Source: CAD feature listing. Evaluate the final solid. Frame: model axes, mm. A direction names the side the tool comes from. Round coordinates to 2 decimals unless told otherwise and drop trailing zeros. Write each loop counter-clockwise with the first axis right and the second up, starting at its lowest first coordinate (ties: lowest second). Pieces come first, ordered by that corner, then holes. Notation, with made-up numbers: M 65.25,71.5 L 108.25,71.5 A27 ccw 108.25,104.5 Z; hole C -29.75,60.25 d5. An arc over 180 degrees is marked long. Answer in a Markdown table with one row per item. Add a question column.
Item 1: Cut plane B-B on z = 96. Return loops of the section in (x, y), and give its area (3 significant figures).
Item 2: Set-up query: faces 1 (the face through (5, 0, 5)), 2 (the face through (-11, 1, 5)), 3 (the face through (-10.95, 5.6, 9.43)). Return all of +Z, -Z, +X, -X, +Y, -Y with unobstructed straight access to the full face (end or side cutting, diameter ignored); none if empty.
Item 3: Cut plane A-A on x = -8. Return loops of the section in (y, z).
Item 4: Mould query, pull axis Y, two halves, no side actions, for faces 4 (the face through (-11, 6.2, 5)), 5 (the face through (-1, 4, 57)), 6 (the face through (-0.57, 12.13, 9.4)). Classes: released by +Y, released by -Y, zero draft, split by the parting line, or undercut.
Item 5: Contact query for flat-ended pins moving along their axis: pin 1 (6 mm diameter, centred on x = -4, z = 49, fed in from -Y); pin 2 (3 mm diameter, centred on x = -10.5, y = 11.5, fed in from +Z); pin 3 (2.5 mm diameter, centred on y = 3.5, z = 81, fed in from -X). Output: stop coordinate, or through.
Item 6: Cut plane C-C on y = -6.75. Return loops of the section in (x, z).
Item 7: Material intervals for probe 1 along Z at (x, y) = (-8, 12.25); probe 2 along X at (y, z) = (5.5, 86); probe 3 along Y at (x, z) = (-4, 59.5), sorted ascending.
Autodesk Inventor part; units mm, degrees
ref_plane "YZ Plane" through (0, 0, 0) normal (1, 0, 0) x (0, 1, 0)
ref_plane "XZ Plane" through (0, 0, 0) normal (0, 1, 0) x (-1, 0, 0)
ref_plane "XY Plane" through (0, 0, 0) normal (0, 0, 1) x (1, 0, 0)
sketch "Esboço1" plane through (0, 0, 0) normal (0, 0, 1) x (1, 0, 0)
  point P0 (0, 0)
sketch "Esboço2" plane through (0, 0, 0) normal (0, 0, 1) x (1, 0, 0)
  line L0 (0, 0) -> (0, 7.2)
  line L1 (0, 7.2) -> (-5.75, 7.2)
  line L2 (-5.75, 7.2) -> (-5.75, 6.2)
  line L3 (-5.75, 6.2) -> (-1, 6.2)
  line L4 (-1, 6.2) -> (-1, 1)
  line L5 (0, 0) -> (-5.75, 0)
  line L6 (-5.75, 0) -> (-5.75, 1)
  line L7 (-5.75, 1) -> (-1, 1)
  dimension "d0" = 7.2
  dimension "d1" = 1
  dimension "d2" = 5.75
  dimension "d3" = 4.75
  dimension "d4" = 5.2
extrude "Extrusão1" add sketch "Esboço2" along normal blind 105
sketch "Esboço3" plane through (-5.75, 0, 0) normal (0, -1, 0) x (1, 0, 0)
  line L0 (5.75, 0) -> (5.75, 105)
  line L1 (5.75, 0) -> (5.75, 10)
  line L2 (5.75, 10) -> (0, 10)
  line L3 (0, 0) -> (0, 105)
  line L4 (0, 10) -> (0, 0)
  line L5 (0, 0) -> (5.75, 0)
  line L6 (0, 0) -> (5.75, 0)
  dimension "d7" = 10
extrude "Extrusão2" add sketch "Esboço3" along normal blind 10
sketch "Esboço4" plane through (0, 0, 105) normal (1, 0, 0) x (0, 0, -1)
  line L0 (105, -10) -> (105, 7.2)
  line L1 (105, 0) -> (105, 7.2)
  line L2 (95, 0) -> (95, -10)
  line L3 (105, 0) -> (95, 0)
  line L4 (95, 0) -> (95, 7.2)
  line L5 (105, 7.2) -> (0, 7.2)
  line L6 (95, 7.2) -> (105, 7.2)
extrude "Extrusão3" add sketch "Esboço4" along normal blind 10
sketch "Esboço5" plane through (-5.75, 7.2, 105) normal (0, 1, 0) x (1, 0, 0)
  line L0 (0, 105) -> (5.75, 105)
  line L1 (0, 105) -> (15.75, 105)
  line L2 (5.75, 105) -> (5.75, 95)
  line L3 (5.75, 95) -> (5.75, 105)
  line L4 (5.75, 95) -> (5.75, 0)
  line L5 (5.75, 105) -> (5.75, 95)
  line L6 (5.75, 95) -> (0, 95)
  line L7 (0, 105) -> (0, 0)
  line L8 (0, 95) -> (0, 105)
extrude "Extrusão4" add sketch "Esboço5" along normal blind 10
sketch "Esboço6" plane through (0, 7.2, 10) normal (1, 0, 0) x (0, 0, -1)
  line L0 (10, -6.2) -> (10, -17.2)
  line L1 (10, -7.2) -> (0, -7.2)
  line L2 (10, -17.2) -> (7, -17.2)
  line L3 (7, -17.2) -> (7, -7.2)
  line L4 (7, -7.2) -> (10, -7.2)
  line L5 (10, -7.2) -> (10, -17.2)
  line L6 (10, -1) -> (10, 10)
  line L7 (10, 10) -> (0, 10)
  line L8 (10, 0) -> (7, 0)
  line L9 (7, 0) -> (7, 10)
  line L10 (7, 10) -> (10, 10)
  line L11 (10, 10) -> (10, 0)
  dimension "d14" = 3
extrude "Extrusão5" add sketch "Esboço6" along normal blind 10
fillet "Arredondamento1" radius 2 4 edges at (5, 7.2, 10) (0, 12.2, 10) (5, 0, 10) (0, -5, 10)
sketch "Esboço7" plane through (-1, 1, 0) normal (-1, 0, 0) x (0, 0, 1)
  line L0 (10, -1) -> (10, -11)
  line L1 (10, 16.2) -> (10, 6.2)
  line L2 (10, -1) -> (10, 6.2)
  line L3 (0, 0) -> (0, -11)
  line L4 (0, 5.2) -> (105, 5.2)
  line L5 (0, 0) -> (10, 0)
  line L6 (10, 0) -> (10, 5.2)
  line L7 (10, 5.2) -> (0, 5.2)
  line L8 (0, 5.2) -> (0, 0)
  point P0 (0, -1)
extrude "Extrusão6" add sketch "Esboço7" along normal blind 15
sketch "Esboço8" plane through (-5.75, 7.2, 10) normal (-1, 0, 0) x (0, 0, 1)
  line L0 (-10, 10) -> (0, 10)
  line L1 (-7, -7.2) -> (-7, -17.2)
  line L2 (-10, 10) -> (-7, 10)
  line L3 (-7, 10) -> (-7, -17.2)
  line L4 (-7, -17.2) -> (-10, -17.2)
  line L5 (-10, -17.2) -> (-10, 10)
  point P0 (-10, -7.2)
extrude "Extrusão7" add sketch "Esboço8" along normal blind 10.25
fillet "Arredondamento2" radius 2 4 edges at (-5.75, 12.2, 10) (-10.875, 6.2, 10) (-10.875, 1, 10) (-5.75, -5, 10)
properties part number "suporte para arma"
Results below:
| question | item | result |
|---|---|---|
| 1 | outline | M -5.75,0 L 0,0 L 0,7.2 L -5.75,7.2 L -5.75,6.2 L -1,6.2 L -1,1 L -5.75,1 Z |
| 1 | area | 16.7 mm2 |
| 2 | face 1 | +Z, +X, -Y |
| 2 | face 2 | +Z, -X, -Y |
| 2 | face 3 | +Z, -X, +Y |
| 3 | outline | M -10,0 L 17.2,0 L 17.2,3 L 6.2,3 L 6.2,8 A2 ccw 4.2,10 L 3,10 A2 ccw 1,8 L 1,3 L -10,3 Z |
| 4 | face 4 | released by +Y |
| 4 | face 5 | undercut |
| 4 | face 6 | zero draft |
| 5 | pin 1 | y = 0 |
| 5 | pin 2 | z = 3 |
| 5 | pin 3 | x = -1 |
| 6 | outline | M -16,0 L 10,0 L 10,3 L 0,3 L 0,8 A2 ccw -2,10 L -3.75,10 A2 ccw -5.75,8 L -5.75,3 L -16,3 Z |
| 7 | probe 1 | 0 to 3 |
| 7 | probe 2 | -1 to 0 |
| 7 | probe 3 | 0 to 1, 6.2 to 7.2 |
